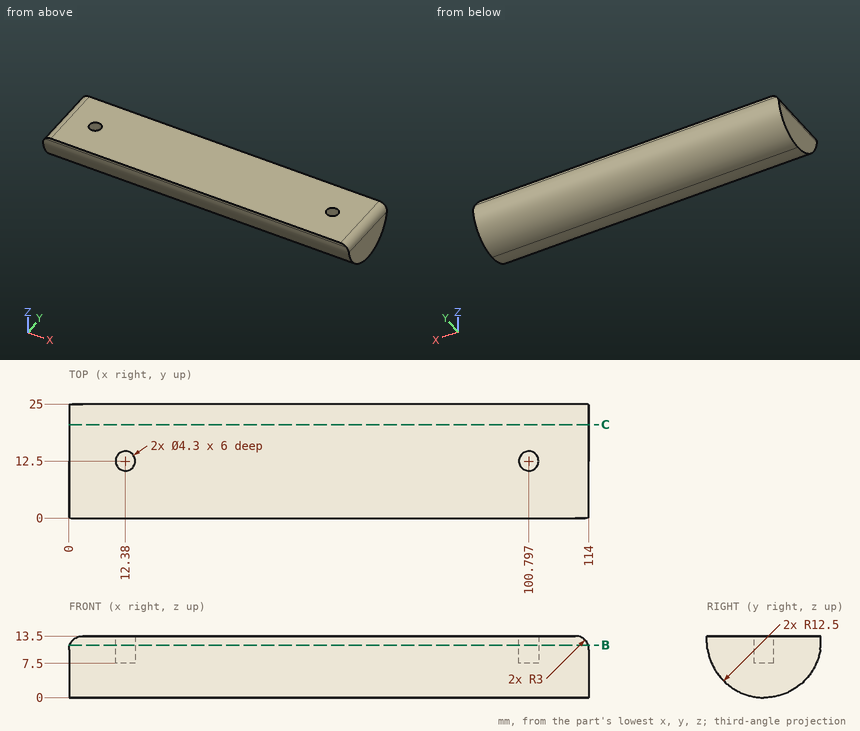
Can you work these out from the drawing? Everything is in mm from the part's minimum corner. Coordinates: 2 decimals unless noted, no trailing zeros. Loops run counter-clockwise (first coordinate to the right, second up) from the corner with the lowest first, then second, coordinate; pieces in that order, holes last.
1) Imagine slicing it at C-C (y = 20.5). List the corners of the cut face in (x, z) for me, and give its area (3 significant figures).
Reported:
outline: (0, 2.9) - (114, 2.9) - (114, 10.5) arc R3 ccw to (111, 13.5) - (3, 13.5) arc R3 ccw to (0, 10.5) - close
area: 1,210 mm2
2) Imagine slicing it at B-B (z = 11.5). List the corners of the cut face in (x, y) for me, and give its area (3 significant figures).
Reported:
outline: (0.17, 0.04) - (113.83, 0.04) - (113.83, 24.96) - (0.17, 24.96) - close; hole circle Ø4.3 at (12.38, 12.5); hole circle Ø4.3 at (100.8, 12.5)
area: 2,800 mm2
3) Please list where these lines run through material, in increasing order: line 1 along X through (y, z) = (10.75, 11.5); line 2 along Y through (x, z) = (43, 12.25); line 3 along Y through (x, z) = (12.38, 10.7).
Reported:
line 1: x = 0.17 to 11.13, 13.63 to 99.55, 102.05 to 113.83
line 2: y = 0 to 25
line 3: y = 0.13 to 10.35, 14.65 to 24.87
4) Will these pins go through, and if not, where does the flat tip stop? pin 1 Ø1 at (x, z) = (38.5, 5.5) entering from +Y; pin 2 Ø2 at (x, z) = (39, 11) entering from +Y; pin 3 Ø1 at (x, y) = (12, 13.5) entering from +Z.
Reported:
pin 1: stops at y = 23.18
pin 2: stops at y = 24.99
pin 3: stops at z = 7.5
